Build history of the part. All positions in model axes, mm. A direction names the side the tool comes from. Give positions to 0.01 mm unless a question says otherwise; leave off trailing zeros. Write each loop counter-clockwise with the first axis right and the second up, starting at its lowest first coordinate (ties: lowest second). Pieces come first, ordered by that corner, then holes. Notation, with made-up numbers: (69.5, 24.25) -> (109.5, 24.25) arc R35 cw to (109.5, 59.25) -> close; hole circle Ø1 at (63.25, 18). An arc over 180 degrees is marked (long way). Write item = value, one per line. Start each with the question number.
Q1. Saw through at A-A, the plane y = 0. List the corners of the cut face in (x, z).
Q2. Saw through at B-B, the plane z = 5.75. List the corners of the cut face in (x, y), then the cut area to 3 significant figures.
Q3. Drop flat-ended pins along their axis: P1, Ø4, axis at x = 1.5, y = -2, coming from the -Z side; P2, Ø8, axis at x = 2.5, y = 2, coming from the -Z side; P3, Ø4, axis at x = -4, y = 4.5, coming from the +Z side; P4, Ø5, axis at y = -3.5, z = 12.5, coming from the -X side. Give the stop position or say it passes through.
Q4. Mould opens along X. For faces 3 (the face through (-0.1, 3.4, 8.5)), 4 (the face through (6.05, 2.82, 1.52)), 5 (the face through (-6.787, -6.748, 4.19)) say: pulls with the +X half, pulls with the -X half, needs draft (parallel to the pull), parting line crosses it, or undercut.
Q5. Saw through at D-D, the plane y = -4.25. List the corners of the cut face in (x, z), then the cut area to 3 significant figures.
Q6. Tool access for faces 1 (the face through (-3.776, -3.749, 1.479)), 2 (the face through (7.5, 0, 4)): list every direction of +Z, -Z, +X, -X, +Y, -Y with a clear straight run to the whole face (end or side of a thin tool).
Q7. Wall check: line 1 (Z direction, x = 4.25, y = -3.75); line 2 (X direction, y = -4.25, z = 2); line 3 (X direction, y = 4, z = 1.5). Give the ranges that are in metal, low to high.
from build123d import *

# Parameters (mm, degrees)
BOSS_EXTRUDE1_DEPTH = 3
FILLET1_R           = 1.5
BOSS_EXTRUDE2_DEPTH = 5.5
SKETCH4_R           = 3.25
BOSS_EXTRUDE3_DEPTH = 11
CHAMFER1_SIZE       = 1


with BuildPart() as part:
    # Sketch1 → Boss-Extrude1 (new body)
    with BuildSketch(Plane.XY):
        with BuildLine():
            Line((5, -7.5), (-5, -7.5))
            ThreePointArc((-5, -7.5), (-6.767766953, -6.767766953), (-7.5, -5))
            Line((-7.5, -5), (-7.5, 5))
            ThreePointArc((-7.5, 5), (-6.767766953, 6.767766953), (-5, 7.5))
            Line((-5, 7.5), (5, 7.5))
            ThreePointArc((5, 7.5), (6.767766953, 6.767766953), (7.5, 5))
            Line((7.5, 5), (7.5, -5))
            ThreePointArc((7.5, -5), (6.767766953, -6.767766953), (5, -7.5))
        make_face()
        with BuildLine():
            Line((3.25, 5), (3.25, 6.5))
            Line((3.25, 6.5), (-5, 6.5))
            ThreePointArc((-5, 6.5), (-6.060660172, 6.060660172), (-6.5, 5))
            Line((-6.5, 5), (-6.5, -3.25))
            Line((-6.5, -3.25), (-5, -3.25))
            ThreePointArc((-5, -3.25), (-3.762563133, -3.762563133), (-3.25, -5))
            Line((-3.25, -5), (-3.25, -6.5))
            Line((-3.25, -6.5), (5, -6.5))
            ThreePointArc((5, -6.5), (6.060660172, -6.060660172), (6.5, -5))
            Line((6.5, -5), (6.5, 3.25))
            Line((6.5, 3.25), (5, 3.25))
            ThreePointArc((5, 3.25), (3.762563133, 3.762563133), (3.25, 5))
        make_face(mode=Mode.SUBTRACT)
    extrude(amount=BOSS_EXTRUDE1_DEPTH)

    # Fillet1
    fillet1_edges = [part.edges().sort_by_distance(p)[0] for p in [
        (-6.5, -3.25, 1.5),
        (-3.25, -6.5, 1.5),
        (6.5, 3.25, 1.5),
        (3.25, 6.5, 1.5),
    ]]
    fillet(fillet1_edges, radius=FILLET1_R - 0.0001)  # a hair under: the kernel refuses the full size

    # Sketch3 → Boss-Extrude2 (add)
    with BuildSketch(Plane.XY.offset(3)):
        with BuildLine():
            Line((-5, -7.5), (5, -7.5))
            ThreePointArc((5, -7.5), (6.767766953, -6.767766953), (7.5, -5))
            Line((7.5, -5), (7.5, 5))
            ThreePointArc((7.5, 5), (6.767766953, 6.767766953), (5, 7.5))
            Line((5, 7.5), (-5, 7.5))
            ThreePointArc((-5, 7.5), (-6.767766953, 6.767766953), (-7.5, 5))
            Line((-7.5, 5), (-7.5, -5))
            ThreePointArc((-7.5, -5), (-6.767766953, -6.767766953), (-5, -7.5))
        make_face()
    extrude(amount=BOSS_EXTRUDE2_DEPTH)

    # Sketch4 → Boss-Extrude3 (add)
    with BuildSketch(Plane.XY.offset(8.5)):
        Circle(SKETCH4_R)
    extrude(amount=BOSS_EXTRUDE3_DEPTH)

    # Chamfer1
    chamfer1_edges = [part.edges().sort_by_distance(p)[0] for p in [
        (-3.25, 0, 19.5),
    ]]
    chamfer(chamfer1_edges, length=CHAMFER1_SIZE)


solid = part.part
Report:
q1.outline = (-7.5, 0) -> (-6.5, 0) -> (-6.5, 3) -> (6.5, 3) -> (6.5, 0) -> (7.5, 0) -> (7.5, 8.5) -> (3.25, 8.5) -> (3.25, 18.5) -> (2.25, 19.5) -> (-2.25, 19.5) -> (-3.25, 18.5) -> (-3.25, 8.5) -> (-7.5, 8.5) -> close
q2.outline = (-7.5, -5) arc R2.5 ccw to (-5, -7.5) -> (5, -7.5) arc R2.5 ccw to (7.5, -5) -> (7.5, 5) arc R2.5 ccw to (5, 7.5) -> (-5, 7.5) arc R2.5 ccw to (-7.5, 5) -> close
q2.area = 220 mm2
q3.P1 = 3
q3.P2 = 0
q3.P3 = 8.5
q3.P4 = -3.09
q4.face_3 = needs draft
q4.face_4 = undercut
q4.face_5 = pulls with the -X half
q5.outline = (-7.5, 0) -> (-3.42, 0) -> (-3.42, 3) -> (6.5, 3) -> (6.5, 0) -> (7.5, 0) -> (7.5, 8.5) -> (-7.5, 8.5) -> close
q5.area = 97.7 mm2
q6.face_1 = -Z
q6.face_2 = +Z, -Z, +X, +Y, -Y
q7.line_1 = 3 to 8.5
q7.line_2 = -7.5 to -3.42, 6.5 to 7.5
q7.line_3 = -7.5 to -6.5, 3.56 to 7.5
